from build123d import *

# Parameters (mm, degrees)
SKETCH1_W               = 19.05
SKETCH1_H               = 19.05
SKETCH1_W_2             = 15.875
SKETCH1_H_2             = 15.875
TUBE_DEPTH              = 539.9532
SKETCH3_R               = 2.8956
REARTOPHOLEMASTER_DEPTH = 20.05
LPATTERN2_COUNT         = 4
LPATTERN2_PITCH         = 142.24


with BuildPart() as part:
    # Sketch1 → Tube (new body)
    with BuildSketch(Plane(origin=(0, 0, 0), x_dir=(0, -1, 0), z_dir=(1, 0, 0))):
        Rectangle(SKETCH1_W, SKETCH1_H)
        Rectangle(SKETCH1_W_2, SKETCH1_H_2, mode=Mode.SUBTRACT)
    extrude(amount=TUBE_DEPTH)

    # Sketch3 → RearTopHoleMaster (cut, through all)
    with BuildSketch(Plane(origin=(0, 9.525, 0), x_dir=(1, 0, 0), z_dir=(0, 1, 0))):
        with Locations((56.6166, 0)):
            Circle(SKETCH3_R)
    reartopholemaster = extrude(amount=-REARTOPHOLEMASTER_DEPTH, mode=Mode.SUBTRACT)

    # LPattern2: RearTopHoleMaster ×4
    with Locations(*[(i * LPATTERN2_PITCH, 0, 0) for i in range(1, LPATTERN2_COUNT)]):
        add(reartopholemaster, mode=Mode.SUBTRACT)


solid = part.part
Geometry: final body of the model. Coordinates: model frame, mm. A direction names the side the tool comes from. Give positions to 0.01 mm unless a question says otherwise; leave off trailing zeros. Write each loop counter-clockwise with the first axis right and the second up, starting at its lowest first coordinate (ties: lowest second). Pieces come first, ordered by that corner, then holes.
(1) Mould query, pull axis Z, two halves, no side actions, for faces 1 (the flat face through (266, 0, -9.525)), 2 (the flat face through (266, 9.525, 0)), 3 (the flat face through (266, 7.938, 0)). Classes: released by +Z, released by -Z, zero draft, split by the parting line, or undercut.
(2) Cut plane A-A, the plane y = 1.5. Return loops of the section in (x, z) (1 decimal), then the cut area to 3 significant figures.
(3) Ray query, line 1 (X direction, y = 8.7, z = 0); line 2 (Y direction, x = 371, z = 1.5) (1 decimal). Return the intervals inside material, ascending.
(4) Cut plane C-C, the plane z = 0. Give the number of separate pieces and of enclosed holes in the cut face, then the cut area to 3 significant figures.
(5) Cut plane B-B, the plane x = 75. Return loops of the section in (y, z) (1 decimal), then the cut area to 3 significant figures.
(6) Access query for faces 4 (the flat face through (266, -7.938, 0)), 5 (the flat face through (0, 9, 0)). Directions: +Z, -Z, +X, -X, +Y, -Y. A direction counts if a zero-diameter tool reaches every point of the face in a straight line with its end or side. Return the directions, or none.
Values follow:
1. face 1: released by -Z
1. face 2: zero draft
1. face 3: undercut
2. outline: (0, -9.5) - (540, -9.5) - (540, -7.9) - (0, -7.9) - close; (0, 7.9) - (540, 7.9) - (540, 9.5) - (0, 9.5) - close
2. area: 1,710 mm2
3. line 1: x = 0 to 53.72, 59.51 to 195.96, 201.75 to 338.2, 343.99 to 480.44, 486.23 to 539.95
3. line 2: y = -9.5 to -7.9, 7.9 to 9.5
4. separate pieces: 10
4. enclosed holes: 0
4. area: 1,640 mm2
5. outline: (-9.5, -9.5) - (9.5, -9.5) - (9.5, 9.5) - (-9.5, 9.5) - close; hole (-7.9, -7.9) - (7.9, -7.9) - (7.9, 7.9) - (-7.9, 7.9) - close
5. area: 111 mm2
6. face 4: +X, -X
6. face 5: +Z, -Z, -X, +Y, -Y
